Geometry check sheet. Reference: the model listing, model coordinates, mm. Give positions to 0.01 mm unless a question says otherwise; leave off trailing zeros. Order: outer loops, then holes, each group sorted by start corner. A loop starts at its lowest first (then second) coordinate and runs counter-clockwise, first axis right, second up. Notation, with made-up numbers: (80, -3.75) - (84, -3.75) arc R13 ccw to (84, 17.25) - close; hole circle Ø5 at (-14.75, -1.75). An arc over 180 degrees is marked (long way). Put each result on its own line as item: value. Start each with the question number.
Autodesk Inventor part; units mm, degrees
ref_plane "Work Plane1" through (5, 0, 0) normal (0, 0, 1) x (1, 0, 0)
ref_plane "YZ Plane" through (0, 0, 0) normal (1, 0, 0) x (0, 1, 0)
ref_plane "XZ Plane" through (0, 0, 0) normal (0, 1, 0) x (-1, 0, 0)
sketch "Skizze1" plane through (0, 0, 0) normal (0, 0, 1) x (1, 0, 0)
  line L0 (0, 0) -> (6.1667, 0)
  line L1 (10, 1.4434) -> (10, 2.5)
  line L2 (10, 2.5) -> (0, 2.5)
  line L3 (10, 1.4434) -> (7, 1.4434)
  line L4 (7, 1.4434) -> (6.1667, 0)
  line L5 (0, -0.5) -> (0, 3)
  line L6 (0, 2.5) -> (0, 0)
  dimension "d0" = 3
  dimension "d1" = 60
  dimension "d2" = 5
  dimension "d3" = 2.8868
  dimension "d5" = 10
revolve "Körper" add sketch "Skizze1" angle 360 about axis through (0, 0, 0) along (1, 0, 0)
sketch "Skizze2" plane through (10, 0, 0) normal (1, 0, 0) x (0, 1, 0)
  circle A0 centre (0, 0) radius 1.4434
  line L0 (-0.7217, 1.25) -> (0.7217, 1.25)
  line L1 (0.7217, 1.25) -> (1.4434, 0)
  line L2 (1.4434, 0) -> (0.7217, -1.25)
  line L3 (0.7217, -1.25) -> (-0.7217, -1.25)
  line L4 (-0.7217, -1.25) -> (-1.4434, 0)
  line L5 (-1.4434, 0) -> (-0.7217, 1.25)
  point P0 (0, 0)
  point P1 (0, 0)
extrude "Loch" add sketch "Skizze2" against normal up to next contours L1 A0 | A0 L2 | L0 A0 | A0 L3 | L5 A0 | A0 L4
thread "Gewinde"
chamfer "Fase1" distance 0.4908 angle 45 1 edges at (10, -2.5, 0) measured on face at (6.6667, 2.4919, -0.2012)
chamfer "Fase2" distance 0.4908 angle 45 1 edges at (0, -2.5, 0) measured on face at (3.1697, 2.4919, -0.2012)
ref_plane "Work Plane1" through (5, 0, 0) normal (0, 0, 1) x (1, 0, 0)
equation "\"d0\" = INTI"
equation "\"d2\" = NND"
equation "\"d3\" = 1.1547 * SW"
equation "\"d5\" = NLG"
equation "\"d8\" = NLG"
equation "\"d10\" = -0.5 * GD1 + 0.5 * NND"
equation "\"d11\" = FAWI"
equation "\"d34\" = -0.5 * GD1 + 0.5 * NND"
equation "\"d12\" = -0.5 * GD1 + 0.5 * NND"
equation "\"d13\" = FAWI"
equation "\"d35\" = -0.5 * GD1 + 0.5 * NND"
equation "\"NND\" = 5"
equation "\"NLG\" = 10"
equation "\"INTI\" = 3"
equation "\"FAWI\" = 45deg"
equation "\"SW\" = 2.5"
equation "\"GD1\" = THREADDIA - 1.2269 * PTC"
equation "\"SPD\" = 3.5"
equation "\"GUL\" = 0.61345 * PTC"
equation "\"TOA\" = 30deg"
equation "\"THREADDIA\" = 5"
equation "\"PTC\" = 0.8"
equation "\"FAWI1\" = 45deg"
equation "\"GAL\" = 0.61345 * PTC"
equation "\"E0\" = 1.155 * SW"
properties part number "DIN 913 - M5 x 10" material "Stahl, weich"
Item 1: Release check for a two-part mould opening along Z. For faces 1 (the face through (6.22, -0.02, -0.09)), 2 (the face through (4.94, -0.54, 2.44)), 3 (the face through (0, 0, 0)) record: +Z half, -Z half, draft (parallel to the pull), parting line (faces both ways), or undercut.
Item 2: Cross-section at B-B (x = 4.25). Enter the section's corners in (y, z), and give its area (3 significant figures).
Item 3: Gauge pin test, flat end, axial feed: pin 1 Ø3 at (x, y) = (9, -1) entering from -Z. Record the tip position at first contact, or that the pin passes through.
Item 4: Thickness scan on line 1 along Z through (x, y) = (8, 0); line 2 along Y through (x, z) = (8.5, 1.1) (3 decimals); line 3 along Z through (x, y) = (9.25, -0.95). Record the ranges inside material, lowest first.
Item 5: Cross-section at A-A (x = 8.5). Enter the section's corners in (y, z), and give its area (3 significant figures).
Recorded:
1. face 1: undercut
1. face 2: parting line
1. face 3: draft
2. outline: circle Ø5 at (0, 0)
2. area: 19.6 mm^2
3. pin 1: stops at z = -2.5
4. line 1: z = -2.5 to -1.25, 1.25 to 2.5
4. line 2: y = -2.245 to -0.808, 0.808 to 2.245
4. line 3: z = -2.31 to -0.85, 0.85 to 2.31
5. outline: circle Ø5 at (0, 0); hole (-1.44, 0) - (-0.72, -1.25) - (0.72, -1.25) - (1.44, 0) - (0.72, 1.25) - (-0.72, 1.25) - close
5. area: 14.2 mm^2
